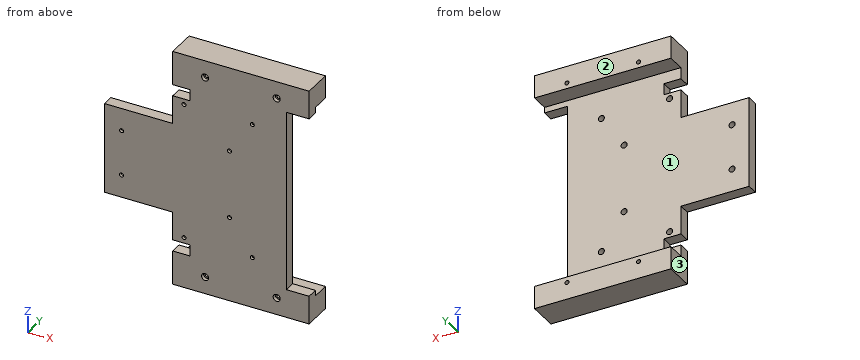
Autodesk Inventor part; units mm, degrees
ref_plane "YZ Plane" through (0, 0, 0) normal (1, 0, 0) x (0, 1, 0)
ref_plane "XZ Plane" through (0, 0, 0) normal (0, 1, 0) x (-1, 0, 0)
ref_plane "XY Plane" through (0, 0, 0) normal (0, 0, 1) x (1, 0, 0)
sketch "Sketch1" plane through (0, 0, 0) normal (0, 1, 0) x (-1, 0, 0)
  line L0 (103.6935, 180.0499) -> (-48.7065, 180.0499)
  line L1 (-48.7065, 180.0499) -> (-48.7065, -86.6501)
  line L2 (-48.7065, -86.6501) -> (103.6935, -86.6501)
  line L3 (103.6935, -86.6501) -> (103.6935, 180.0499)
  point P0 (0, 0)
  dimension "d0" = 266.7
  dimension "d1" = 152.4
extrude "Extrusion1" add sketch "Sketch1" along normal blind 12.7
sketch "Sketch2" plane through (0, 12.7, 0) normal (0, 1, 0) x (1, 0, 0)
  line L0 (-103.6935, 86.6501) -> (-103.6935, -180.0499)
  line L1 (-103.6935, -180.0499) -> (48.7065, -180.0499)
  line L2 (48.7065, -180.0499) -> (48.7065, -154.6499)
  line L3 (48.7065, -154.6499) -> (-103.6935, -154.6499)
  line L4 (-103.6935, -154.6499) -> (-103.6935, -180.0499)
  line L5 (48.7065, -180.0499) -> (48.7065, 86.6501)
  line L6 (48.7065, 86.6501) -> (-103.6935, 86.6501)
  line L7 (-103.6935, 86.6501) -> (-103.6935, 61.2501)
  line L8 (-103.6935, 61.2501) -> (48.7065, 61.2501)
  line L9 (48.7065, 61.2501) -> (48.7065, 86.6501)
  point P0 (0, 0)
  dimension "d4" = 25.4
  dimension "d5" = 25.4
  dimension "d8" = 0
extrude "Extrusion2" add sketch "Sketch2" along normal blind 20.1422 contours L6 L5 L8 L0 | L3 L2 L1 L0
sketch "Sketch3" plane through (0, 0, 0) normal (0, -1, 0) x (1, 0, 0)
  line L0 (94.7395, 46.6999) -> (-172.7542, 46.6999)
  line L1 (-103.6935, 180.0499) -> (48.7065, 180.0499)
  line L2 (-27.4935, 259.5672) -> (-27.4935, -153.6047)
  line L3 (48.7065, 180.0499) -> (48.7065, -86.6501)
  point P0 (0, 0)
  point P1 (12.5115, 160.9999)
  point P2 (-67.4985, 160.9999)
  point P3 (12.5115, -67.6001)
  point P4 (-67.4985, -67.6001)
  dimension "d9" = 133.35
  dimension "d10" = 76.2
  dimension "d11" = 40.005
  dimension "d12" = 40.005
  dimension "d13" = 0
  dimension "d14" = 0
  dimension "d15" = 114.3
  dimension "d16" = 0
  dimension "d17" = 0
  dimension "d18" = 114.3
hole "Hole1" at (12.5115, 0, 160.9999) at (-67.4985, 0, 160.9999) at (12.5115, 0, -67.6001) at (-67.4985, 0, -67.6001) direction (0, 1, 0) diameter 4.4958 end through all counterbore diameter 7.9502 counterbore depth 4.1656
sketch "Sketch4" plane through (-103.6935, 0, -86.6501) normal (-1, 0, 0) x (0, 0, 1)
  line L0 (184.15, 0) -> (82.55, 0)
  line L1 (82.55, 0) -> (82.55, 12.7)
  line L2 (82.55, 12.7) -> (184.15, 12.7)
  line L3 (184.15, 12.7) -> (184.15, 0)
  line L4 (0, 0) -> (0, 32.8422)
  line L5 (0, 0) -> (266.7, 0)
  line L6 (25.4, 12.7) -> (241.3, 12.7)
  line L7 (266.7, 0) -> (266.7, 32.8422)
  point P0 (86.6501, 0)
  dimension "d26" = 101.6
  dimension "d27" = 82.55
  dimension "d28" = 0
  dimension "d29" = 0
  dimension "d53" = 82.55
extrude "Extrusion3" add sketch "Sketch4" along normal blind 76.2
sketch "Sketch5" plane through (0, 0, 0) normal (0, -1, 0) x (1, 0, 0)
  line L0 (-103.6935, 97.4999) -> (-179.8935, 97.4999)
  line L1 (-103.6935, -4.1001) -> (-179.8935, -4.1001)
  line L2 (48.7065, 180.0499) -> (48.7065, -86.6501)
  line L3 (-103.6935, -86.6501) -> (-103.6935, -4.1001)
  point P0 (0, 0)
  point P1 (-14.7935, 122.8999)
  point P2 (-90.9935, 122.8999)
  point P3 (-90.9935, -29.5001)
  point P4 (-14.7935, -29.5001)
  dimension "d32" = 0
  dimension "d33" = 0
  dimension "d34" = 25.4
  dimension "d35" = 25.4
  dimension "d36" = 0
  dimension "d38" = 12.7
  dimension "d52" = 76.2
  dimension "d54" = 0
hole "Hole2" at (-14.7935, 0, 122.8999) at (-90.9935, 0, 122.8999) at (-90.9935, 0, -29.5001) at (-14.7935, 0, -29.5001) direction (0, 1, 0) diameter 4.4958 end through all
sketch "Sketch6" plane through (0, 12.7, 0) normal (0, 1, 0) x (1, 0, 0)
  circle A0 centre (-90.9935, -122.8999) radius 2.2479
  circle A1 centre (-14.7935, -122.8999) radius 2.2479
  circle A2 centre (-14.7935, 29.5001) radius 2.2479
  circle A3 centre (-90.9935, 29.5001) radius 2.2479
  circle A4 centre (-90.9935, 29.5001) radius 2.2479
  circle A5 centre (-90.9935, 29.5001) radius 3.3734
  circle A6 centre (-90.9935, -122.8999) radius 3.3734
  circle A7 centre (-14.7935, -122.8999) radius 3.3734
  circle A8 centre (-14.7935, 29.5001) radius 3.3734
  point P0 (0, 0)
  dimension "d46" = 6.7469
  dimension "d47" = 6.7469
  dimension "d48" = 6.7469
  dimension "d49" = 6.7469
extrude "Extrusion4" cut sketch "Sketch6" against normal blind 9.525 contours A0 | A1 | A2 | A3 | A5 | A6 | A7 | A8
sketch "Sketch7" plane through (0, 0, 0) normal (0, -1, 0) x (1, 0, 0)
  line L0 (85.2483, 148.2999) -> (23.3065, 148.2999)
  line L1 (23.3065, 148.2999) -> (23.3065, -54.9001)
  line L2 (23.3065, -54.9001) -> (85.2483, -54.9001)
  line L3 (85.2483, -54.9001) -> (85.2483, 148.2999)
  line L4 (48.7065, -86.6501) -> (-103.6935, -86.6501)
  line L5 (-103.6935, 180.0499) -> (48.7065, 180.0499)
  line L6 (48.7065, 180.0499) -> (48.7065, -86.6501)
  point P0 (0, 0)
  dimension "d55" = 31.75
  dimension "d56" = 31.75
  dimension "d57" = 25.4
extrude "Extrusion5" cut sketch "Sketch7" against normal blind 50.8
sketch "Sketch8" plane through (0, 0, 0) normal (0, -1, 0) x (1, 0, 0)
  line L0 (-111.6685, 129.2499) -> (-84.6435, 129.2499)
  line L1 (-84.6435, 129.2499) -> (-84.6435, 141.9499)
  line L2 (-84.6435, 141.9499) -> (-111.6685, 141.9499)
  line L3 (-111.6685, 141.9499) -> (-111.6685, 129.2499)
  line L4 (-115.7126, -48.5501) -> (-84.6435, -48.5501)
  line L5 (-84.6435, -48.5501) -> (-84.6435, -35.8501)
  line L6 (-84.6435, -35.8501) -> (-115.7126, -35.8501)
  line L7 (-115.7126, -35.8501) -> (-115.7126, -48.5501)
  line L8 (-103.6935, -86.6501) -> (-103.6935, -4.1001)
  line L9 (-103.6935, 97.4999) -> (-103.6935, 180.0499)
  point P0 (0, 0)
  point P1 (-103.6935, -61.2501)
  point P2 (-103.6935, 154.6499)
  dimension "d60" = 12.7
  dimension "d61" = 12.7
  dimension "d62" = 19.05
  dimension "d63" = 19.05
  dimension "d64" = 12.7
  dimension "d65" = 12.7
extrude "Extrusion6" cut sketch "Sketch8" against normal blind 50.8
sketch "Sketch9" plane through (0, 0, 0) normal (0, -1, 0) x (1, 0, 0)
  line L0 (-103.6935, 180.0499) -> (48.7065, 180.0499)
  line L1 (48.7065, 180.0499) -> (48.7065, 148.2999)
  point P0 (0, 0)
  point P1 (-40.1935, 84.7999)
  point P2 (-40.1935, 8.5999)
  dimension "d68" = 76.2
  dimension "d69" = 0
  dimension "d70" = 95.25
  dimension "d71" = 88.9
hole "Hole3" at (-40.1935, 0, 84.7999) at (-40.1935, 0, 8.5999) direction (0, 1, 0) diameter 4.4958 end through all
sketch "Sketch10" plane through (0, 12.7, 0) normal (0, 1, 0) x (1, 0, 0)
  circle A0 centre (-40.1935, -84.7999) radius 2.2479
  circle A1 centre (-40.1935, -8.5999) radius 2.2479
  circle A2 centre (-40.1935, -8.5999) radius 2.2479
  circle A3 centre (-40.1935, -8.5999) radius 3.3734
  circle A4 centre (-40.1935, -84.7999) radius 3.3734
  point P0 (0, 0)
  dimension "d79" = 6.7469
  dimension "d80" = 6.7469
extrude "Extrusion7" cut sketch "Sketch10" against normal blind 9.525 contours A0 | A1 | A3 | A4
sketch "Sketch11" plane through (0, 0, 0) normal (0, -1, 0) x (1, 0, 0)
  circle A0 centre (-40.1935, 8.5999) radius 2.2479
  point P0 (0, 0)
  point P1 (-160.8435, 21.2999)
  point P2 (-160.8435, 72.0999)
  dimension "d83" = 120.65
  dimension "d84" = 0
  dimension "d85" = 50.8
  dimension "d86" = 12.7
hole "Hole4" at (-160.8435, 0, 21.2999) at (-160.8435, 0, 72.0999) direction (0, 1, 0) diameter 4.4958 end through all
sketch "Sketch12" plane through (0, 12.7, 0) normal (0, 1, 0) x (1, 0, 0)
  circle A0 centre (-160.8435, -72.0999) radius 2.2479
  circle A1 centre (-160.8435, -21.2999) radius 2.2479
  circle A2 centre (-160.8435, -21.2999) radius 3.3734
  circle A3 centre (-160.8435, -72.0999) radius 3.3734
  point P0 (0, 0)
  dimension "d94" = 6.7469
  dimension "d95" = 6.7469
extrude "Extrusion8" cut sketch "Sketch12" against normal blind 9.525 contours A0 | A1 | A2 | A3
properties part number "MotorPlate"
Build history of the part. All positions in model axes, mm. Face numbers are marked on the shaded views. A direction names the side the tool comes from. Round coordinates to 2 decimals unless told otherwise and drop trailing zeros. Write each loop counter-clockwise with the first axis right and the second up, starting at its lowest first coordinate (ties: lowest second). Pieces come first, ordered by that corner, then holes. Notation, with made-up numbers: (68.5, -11.75) -> (119.5, -11.75) arc R24 cw to (119.5, 7.25) -> close; hole circle Ø10 at (50, 19). An arc over 180 degrees is marked (long way). Put each result on its own line as item: value.
Item 1: Slice it at C-C, the plane y = 9. Count the separate pieces of the cut face and the enclosed holes in it, plus the area to 3 significant figures.
Here are the results:
separate pieces: 1
enclosed holes: 12
area: 42,400 mm^2
Item 2: Slice it at A-A, the plane x = 33.5. Give the cut face in (y, z).
Here are the results:
outline: (0, -86.65) -> (32.84, -86.65) -> (32.84, -61.25) -> (12.7, -61.25) -> (12.7, -54.9) -> (0, -54.9) -> close; (0, 148.3) -> (12.7, 148.3) -> (12.7, 154.65) -> (32.84, 154.65) -> (32.84, 180.05) -> (0, 180.05) -> close
Item 3: Flat gauge pins, fed straight in: P1, Ø3.5, axis at x = -160.84, z = 72.1, coming from the +Y side; P2, Ø6, axis at x = -126.5, y = 14, coming from the -Z side; P3, Ø1.5, axis at x = -90.5, z = -25, coming from the +Y side; P4, Ø3.5, axis at x = -91, z = -30.5, coming from the +Y side (3 decimals). Where does each tip first touch, or does it go through?
Here are the results:
P1: passes through
P2: stops at z = -4.1
P3: stops at y = 12.7
P4: stops at y = 3.175
Item 4: Wall check: probe 1 along Z at (x, y) = (-52, 25.5); probe 2 along X at (y, z) = (2, -66); probe 3 along Y at (x, z) = (-23, 108.5). Give the ranges that are in metal, low to high. Write a range as from..to.
Here are the results:
probe 1: z = -86.65..-61.25, 154.65..180.05
probe 2: x = -103.69..-71.14, -63.86..8.87, 16.15..48.71
probe 3: y = 0..12.7
Item 5: Slice it at B-B, the plane y = 24. Give the cut face in (x, z), plus the area to 3 significant figures.
Here are the results:
outline: (-103.69, -86.65) -> (48.71, -86.65) -> (48.71, -61.25) -> (-103.69, -61.25) -> close; (-103.69, 154.65) -> (48.71, 154.65) -> (48.71, 180.05) -> (-103.69, 180.05) -> close; hole circle Ø4.5 at (-67.5, -67.6); hole circle Ø4.5 at (-67.5, 161); hole circle Ø4.5 at (12.51, -67.6); hole circle Ø4.5 at (12.51, 161)
area: 7,680 mm^2
Item 6: Slice it at D-D, the plane x = -27.5. Give the cut face in (y, z), plus the area to 3 significant figures.
Here are the results:
outline: (0, -86.65) -> (32.84, -86.65) -> (32.84, -61.25) -> (12.7, -61.25) -> (12.7, 154.65) -> (32.84, 154.65) -> (32.84, 180.05) -> (0, 180.05) -> close
area: 4,410 mm^2
Item 7: Tool access for the marked faces 1, 2 and 3: list every direction of +Z, -Z, +X, -X, +Y, -Y with a clear straight run to the whole face (end or side of a thin tool).
Here are the results:
face 1: +X, -X, +Y
face 2: +Z, -Z, +X, -X, +Y
face 3: -Z, -X, +Y, -Y
